from build123d import *

# Parameters (mm, degrees)
CUT_EXTRUDE1_DEPTH = 0.5
CIRPATTERN1_COUNT  = 4


with BuildPart() as part:
    # Sketch1 → Revolve1 (revolve)
    with BuildSketch(Plane.XY, mode=Mode.PRIVATE) as revolve1_sk:
        Polygon((-1.5, 0), (-1.5, -10), (0, -10), (0, 1.375), (-2.875, 1.375), align=None)
    revolve(revolve1_sk.sketch.rotate(Axis((0, 0, 0), (0, -1, 0)), 270), axis=Axis((0, 0, 0), (0, -1, 0)))

    # Sketch2 → Cut-Extrude1 (cut, symmetric)
    with BuildSketch(Plane.XY):
        Polygon((-2.11777299, 1.375), (2.11777299, 1.375), (0.472629215, 0.516963183), (-0.472629215, 0.516963183), align=None)
    cut_extrude1 = extrude(amount=CUT_EXTRUDE1_DEPTH, both=True, mode=Mode.SUBTRACT)

    # CirPattern1: Cut-Extrude1 ×4 about axis
    cirpattern1_axis = Axis((0, 0, 0), (0, 1, 0))
    for i in range(1, CIRPATTERN1_COUNT):
        add(cut_extrude1.rotate(cirpattern1_axis, i * 360 / CIRPATTERN1_COUNT), mode=Mode.SUBTRACT)


solid = part.part
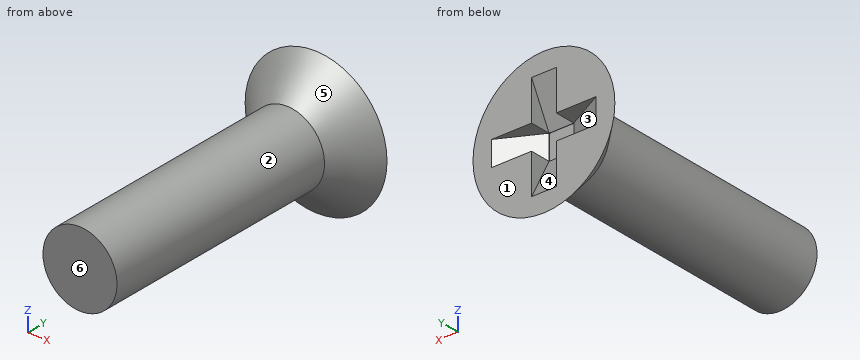
Work out the finished part from the listing and answer in its coordinate system (mm). Face numbers are marked on the shaded views. A direction names the side the tool comes from. Give positions to 0.01 mm unless a question says otherwise; leave off trailing zeros. Loops run counter-clockwise (first coordinate to the right, second up) from the corner with the lowest first, then second, coordinate; pieces in that order, holes last. Notation, with made-up numbers: (20, -10.5) - (40, -10.5) arc R23 ccw to (40, 4.5) - close; hole circle Ø2 at (48, 78.25). An arc over 180 degrees is marked (long way). Answer in a Markdown table with one row per item. Add a question column.
Q1. The part is cut by section C-C (y = -5.75). Determine the outline of the cut face in (x, z), and give its area (3 significant figures).
Q2. The part is cut by section B-B (x = 0). Determine the outline of the cut face in (y, z) (3 decimals).
Q3. A tool of negligible diameter and unlimited length cuts with its end or side. For the marked faces 1, 2 and 3, from which of +Z, -Z, +X, -X, +Y, -Y can it reach the whole face along a straight path? Write none if from no direction.
Q4. Determine the mould class of the marked faces 4, 5 and 6 for opening direction Z: released by +Z, released by -Z, zero draft, split by the parting line, or undercut.
Q5. The part is cut by section A-A (z = 0). Determine the outline of the cut face in (x, y) (3 decimals), and give its area (3 significant figures).
Q6. Consider line 1 along X through (y, z) = (-7.5, -1.1); line 2 along Y through (x, z) = (0.3, 0.1); line 3 along X through (y, z) = (-6.25, 0.45). Determine where each line is inside the solid, lowest interval first.
Q7. Each of these flat-tipped pins is pushed along its axis until it touches: P1, Ø1.1, axis at x = 0, z = 0, coming from the +Y side; P2, Ø0.7, axis at y = 1, z = -1, coming from the +X side; P3, Ø0.7, axis at x = -1.5, y = 1, coming from the -Z side. Where does it stop, or does it pass through?
Solution:
| question | item | result |
|---|---|---|
| 1 | outline | circle Ø3 at (0, 0) |
| 1 | area | 7.07 mm² |
| 2 | outline | (-10, -1.5) - (0, -1.5) - (1.375, -2.875) - (1.375, -2.118) - (0.531, -0.5) - (0.517, -0.5) - (0.517, 0.5) - (0.531, 0.5) - (1.375, 2.118) - (1.375, 2.875) - (0, 1.5) - (-10, 1.5) - close |
| 3 | face 1 | +Z, -Z, +X, -X, +Y |
| 3 | face 2 | -Y |
| 3 | face 3 | +Y |
| 4 | face 4 | undercut |
| 4 | face 5 | split by the parting line |
| 4 | face 6 | zero draft |
| 5 | outline | (-2.875, 1.375) - (-1.5, 0) - (-1.5, -10) - (1.5, -10) - (1.5, 0) - (2.875, 1.375) - (2.118, 1.375) - (0.5, 0.531) - (0.5, 0.517) - (-0.5, 0.517) - (-0.5, 0.531) - (-2.118, 1.375) - close |
| 5 | area | 33.8 mm² |
| 6 | line 1 | x = -1.02 to 1.02 |
| 6 | line 2 | y = -10 to 0.52 |
| 6 | line 3 | x = -1.43 to 1.43 |
| 7 | P1 | stops at y = 0.56 |
| 7 | P2 | stops at x = 2.69 |
| 7 | P3 | stops at z = -2.47 |
